Build history of the part. All positions in model axes, mm. A direction names the side the tool comes from. Round coordinates to 2 decimals unless told otherwise and drop trailing zeros. Loops run counter-clockwise (first coordinate to the right, second up) from the corner with the lowest first, then second, coordinate; pieces in that order, holes last. Notation, with made-up numbers: M 80,-2.75 L 103,-2.75 A32 cw 103,34.25 Z; hole C 61,16 d11. An arc over 180 degrees is marked long. One line per item, written item: value.
```python
from build123d import *

# Parameters (mm, degrees)
BOSS_EXTRUDE2_DEPTH = 6.35
SKETCH3_W           = 30.1625
SKETCH3_H           = 11.1125
CUT_EXTRUDE1_DEPTH  = 6.35


with BuildPart() as part:
    # Sketch1 → Boss-Extrude2 (new body)
    with BuildSketch(Plane(origin=(0, 0, 0), x_dir=(1, 0, 0), z_dir=(0, 1, 0))):
        Polygon((114.3, 95.25), (85.725, 95.25), (85.725, 88.9), (28.575, 88.9), (28.575, 95.25), (-28.575, 95.25), (-28.575, 88.9), (-85.725, 88.9), (-85.725, 95.25), (-114.3, 95.25), (-114.3, 88.9), (-107.95, 88.9), (-107.95, 79.375), (-114.3, 79.375), (-114.3, 47.625), (-107.95, 47.625), (-107.95, 15.875), (-114.3, 15.875), (-114.3, -15.875), (-107.95, -15.875), (-107.95, -47.625), (-114.3, -47.625), (-114.3, -79.375), (-107.95, -79.375), (-107.95, -88.9), (-114.3, -88.9), (-114.3, -95.25), (-85.725, -95.25), (-85.725, -88.9), (-28.575, -88.9), (-28.575, -95.25), (28.575, -95.25), (28.575, -88.9), (85.725, -88.9), (85.725, -95.25), (114.3, -95.25), (114.3, -88.9), (107.95, -88.9), (107.95, -79.375), (114.3, -79.375), (114.3, -47.625), (107.95, -47.625), (107.95, -15.875), (114.3, -15.875), (114.3, 15.875), (107.95, 15.875), (107.95, 47.625), (114.3, 47.625), (114.3, 79.375), (107.95, 79.375), (107.95, 88.9), (114.3, 88.9), align=None)
    extrude(amount=BOSS_EXTRUDE2_DEPTH)

    # Sketch3 → Cut-Extrude1 (cut)
    with BuildSketch(Plane(origin=(0, 6.35, 0), x_dir=(1, 0, 0), z_dir=(0, 1, 0))):
        with Locations((78.868959442, -66.665058112)):
            Rectangle(SKETCH3_W, SKETCH3_H)
    extrude(amount=-CUT_EXTRUDE1_DEPTH, mode=Mode.SUBTRACT)


solid = part.part
```
Item 1: Pull direction X, two halves, no side cores. Call faces 5 (the face through (-58, 3, 88.9)), 6 (the face through (111, 3, -79.375)), 7 (the face through (-57, 3, -88.9)), 8 (the face through (107.95, 3, -84)): pulls with the +X half, pulls with the -X half, needs draft (parallel to the pull), parting line crosses it, or undercut.
Check values:
face 5: undercut
face 6: needs draft
face 7: undercut
face 8: pulls with the +X half
Item 2: Wall check: line 1 along Z through (x, y) = (76.5, 2.5); line 2 along X through (y, z) = (3.5, 64); line 3 along X through (y, z) = (0.75, 27). Give the ranges that are in metal, low to high.
Check values:
line 1: z = -88.9 to 61.11, 72.22 to 88.9
line 2: x = -114.3 to 63.79, 93.95 to 114.3
line 3: x = -107.95 to 107.95
Item 3: Drop flat-ended pins along their axis: P1, Ø3, axis at y = 4, z = 82.5, coming from the -X side; P2, Ø3, axis at x = -45, y = 5, coming from the +Z side. Give the stop position or say it passes through.
Check values:
P1: stops at x = -107.95
P2: stops at z = 88.9
Item 4: Slice it at A-A, the plane z = 31.5. Give the cut face in (x, y).
Check values:
outline: M -107.95,0 L 107.95,0 L 107.95,6.35 L -107.95,6.35 Z
Item 5: Which spindle directions (+Z, -Z, +X, -X, +Y, -Y) get a long thin tool onto all of the face, cutting with end or side? Do faces 1 (the face through (79, 3, 72.221)), 2 (the face through (-28.575, 3, -92)), 3 (the face through (85.725, 3, 92)), 4 (the face through (-107.95, 3, 32)). Say none if no direction does.
Check values:
face 1: +Y, -Y
face 2: -Z, +Y, -Y
face 3: +Z, +Y, -Y
face 4: -X, +Y, -Y
Item 6: Slice it at B-B, the plane x = -43. Give the cut face in (y, z).
Check values:
outline: M 0,-88.9 L 6.35,-88.9 L 6.35,88.9 L 0,88.9 Z
